Verification items for the finished model (mm, model axes). Face numbers are marked on the shaded views. Give positions to 0.01 mm unless a question says otherwise; leave off trailing zeros. Loops run counter-clockwise (first coordinate to the right, second up) from the corner with the lowest first, then second, coordinate; pieces in that order, holes last. Notation, with made-up numbers: (-11.75, -18.5) -> (7.25, -18.5) arc R17 ccw to (7.25, -8.5) -> close; hole circle Ø7 at (83.5, 16). An arc over 180 degrees is marked (long way). Answer in a Markdown table with one row per item. Add a question column.
Q1. Gauge pin test, flat ends, axial feed: P1, Ø2, axis at x = 7, y = 25.5, coming from the +Z side; P2, Ø8, axis at x = -16, y = 19, coming from the +Z side; P3, Ø1, axis at y = 20.5, z = 36, coming from the +X side. Record the tip position at first contact, or that the pin passes through.
Q2. Material ranges on probe 1 along Y at (x, z) = (27, 8.5); probe 2 along X at (y, z) = (31.5, 42); probe 3 along Y at (x, z) = (-15.5, 50), recorded low to high.
Q3. Release check for a two-part mould opening along X. For the marked faces 1 and 2 record: pulls with the +X half, pulls with the -X half, needs draft (parallel to the pull), parting line crosses it, or undercut.
Q4. Section check A-A on x = 0. Enter the section's corners in (y, z), and give its area (3 significant figures).
Q5. Section check B-B on z = 58. Enter the section's corners in (x, y).
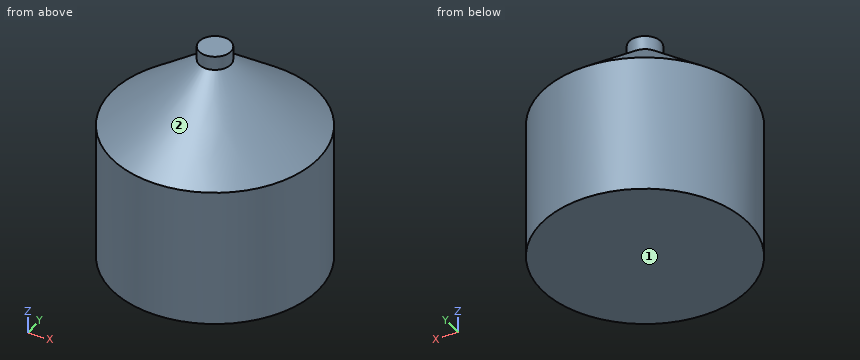
```python
from build123d import *

# Parameters (mm, degrees)
F0_R      = 37.3463953666
F1_DEPTH  = 50
F1_FACE_R = 37.3463953666
F3_R      = 5.7348766561
F5_DEPTH  = 5


with BuildPart() as f1:
    # F0 (on Top) → F1 (new body)
    with BuildSketch(Plane.XY):
        Circle(F0_R)
    extrude(amount=F1_DEPTH)

    # F1_face (on face) → F4 section 0
    with BuildSketch(Plane.XY.offset(50)):
        Circle(F1_FACE_R)
    # F3 (on offset) → F4 section 1
    with BuildSketch(Plane.XY.offset(75)):
        Circle(F3_R)
    loft()

    # F5 (add): a face of the model
    f5_faces = [f1.faces().sort_by_distance(p)[0] for p in [
        (0, 0, 75),
    ]]
    extrude(f5_faces, amount=F5_DEPTH)


solid = f1.part
```
Taken from the geometry:
| question | item | result |
|---|---|---|
| 1 | P1 | stops at z = 59.41 |
| 1 | P2 | stops at z = 63.05 |
| 1 | P3 | stops at x = 31.54 |
| 2 | probe 1 | y = -25.8 to 25.8 |
| 2 | probe 2 | x = -20.06 to 20.06 |
| 2 | probe 3 | y = -33.98 to 33.98 |
| 3 | face 1 | needs draft |
| 3 | face 2 | parting line crosses it |
| 4 | outline | (-37.35, 0) -> (37.35, 0) -> (37.35, 50) -> (5.73, 75) -> (5.73, 80) -> (-5.73, 80) -> (-5.73, 75) -> (-37.35, 50) -> close |
| 4 | area | 4,870 mm² |
| 5 | outline | circle Ø54.46 at (0, 0) |
